Work out the finished part from the listing and answer in its coordinate system (mm). Coordinates: 2 decimals unless noted, no trailing zeros. Write each loop counter-clockwise with the first axis right and the second up, starting at its lowest first coordinate (ties: lowest second). Pieces come first, ordered by that corner, then holes. Notation, with made-up numbers: (69, -35.75) -> (103, -35.75) arc R16 cw to (103, -25.75) -> close; hole circle Ø6 at (47.5, 10). An arc over 180 degrees is marked (long way). Write each question's results on one line, items separated by ' | '. Start each with the question number.
from build123d import *

# Parameters (mm, degrees)
CROQUIS1_R              = 1.5
CROQUIS1_W              = 44
CROQUIS1_H              = 26
CROQUIS1_W_2            = 5
CROQUIS1_H_2            = 26.666666666
CROQUIS1_W_3            = 76.666666666
CROQUIS1_H_3            = 5
SALIENTE_EXTRUIR1_DEPTH = 5
CROQUIS2_R              = 4.15
CORTAR_EXTRUIR1_DEPTH   = 10
CROQUIS3_W              = 19
CROQUIS3_H              = 13
CORTAR_EXTRUIR2_DEPTH   = 10
CROQUIS4_R              = 4.15
CORTAR_EXTRUIR3_DEPTH   = 10
CROQUIS5_R              = 6
CORTAR_EXTRUIR4_DEPTH   = 10
CROQUIS7_W              = 87.958060954
CROQUIS7_H              = 14.714173765
SALIENTE_EXTRUIR2_DEPTH = 5


with BuildPart() as part:
    # Croquis1 → Saliente-Extruir1 (new body)
    with BuildSketch(Plane.XY):
        Polygon((5, 26.666666667), (5, 5), (76.666666667, 5), (153.333333333, 5), (225, 5), (225, 26.666666667), (225, 53.333333333), (225, 75), (153.333333333, 75), (76.666666667, 75), (5, 75), (5, 53.333333333), align=None)
        with Locations((30, 39)):
            Circle(CROQUIS1_R, mode=Mode.SUBTRACT)
        with Locations((83.04, 39)):
            Circle(CROQUIS1_R, mode=Mode.SUBTRACT)
        with Locations((56.52, 52)):
            Rectangle(CROQUIS1_W, CROQUIS1_H, mode=Mode.SUBTRACT)
        with Locations((30, 65)):
            Circle(CROQUIS1_R, mode=Mode.SUBTRACT)
        with Locations((83.04, 65)):
            Circle(CROQUIS1_R, mode=Mode.SUBTRACT)
        with Locations((227.5, 40)):
            Rectangle(CROQUIS1_W_2, CROQUIS1_H_2)
        with Locations((115, 2.5)):
            Rectangle(CROQUIS1_W_3, CROQUIS1_H_3)
        with Locations((2.5, 40)):
            Rectangle(CROQUIS1_W_2, CROQUIS1_H_2)
        with Locations((115, 77.5)):
            Rectangle(CROQUIS1_W_3, CROQUIS1_H_3)
    extrude(amount=SALIENTE_EXTRUIR1_DEPTH)

    # Croquis2 → Cortar-Extruir1 (cut)
    with BuildSketch(Plane.XY.offset(5)):
        with Locations((96.666666667, 20)):
            Circle(CROQUIS2_R)
        with Locations((116.666666667, 20)):
            Circle(CROQUIS2_R)
        with Locations((136.666666667, 20)):
            Circle(CROQUIS2_R)
    extrude(amount=-CORTAR_EXTRUIR1_DEPTH, mode=Mode.SUBTRACT)

    # Croquis3 → Cortar-Extruir2 (cut)
    with BuildSketch(Plane.XY.offset(5)):
        with Locations((34.5, 20.5)):
            Rectangle(CROQUIS3_W, CROQUIS3_H)
    extrude(amount=-CORTAR_EXTRUIR2_DEPTH, mode=Mode.SUBTRACT)

    # Croquis4 → Cortar-Extruir3 (cut)
    with BuildSketch(Plane.XY.offset(5)):
        with Locations((65, 20)):
            Circle(CROQUIS4_R)
        with Locations((80, 20)):
            Circle(CROQUIS4_R)
    extrude(amount=-CORTAR_EXTRUIR3_DEPTH, mode=Mode.SUBTRACT)

    # Croquis5 → Cortar-Extruir4 (cut)
    with BuildSketch(Plane.XY.offset(5)):
        with Locations((98.52, 50)):
            Circle(CROQUIS5_R)
        with Locations((120.52, 50)):
            Circle(CROQUIS5_R)
    extrude(amount=-CORTAR_EXTRUIR4_DEPTH, mode=Mode.SUBTRACT)

    # Croquis7 → Saliente-Extruir2 (add)
    with BuildSketch(Plane.XY.offset(5)):
        with Locations((100.697748768, 19.971943706)):
            Rectangle(CROQUIS7_W, CROQUIS7_H)
    extrude(amount=-SALIENTE_EXTRUIR2_DEPTH)


solid = part.part
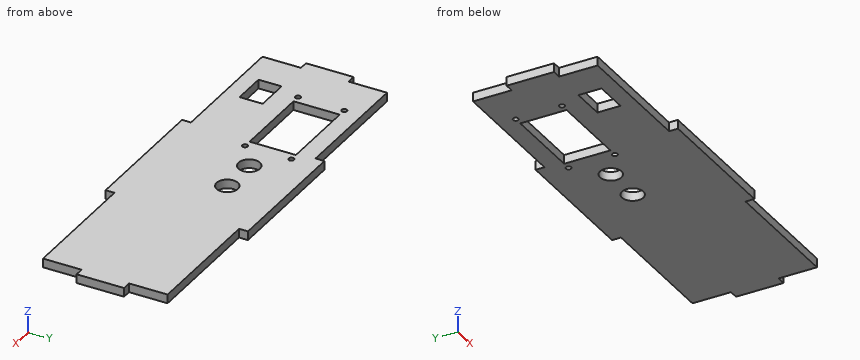
1. Find section A-A on x = 98.52. Give the vertices of the cut face in (y, z).
2. Find section C-C on x = 41.5. Give the vertices of the cut face in (y, z), and give its area (3 significant figures).
3. Given pin 1 Ø2.5 at (x, y) = (30, 65) entering from -Z; pin 2 Ø1.5 at (y, z) = (3, 1.5) entering from -X; pin 3 Ø1.5 at (y, z) = (20.5, 3.5) entering from -X; pin 4 Ø19 at (x, y) = (120.52, 50) entering from +Z, each flat-ended and moving along its own axis, determine where each tip first touches the part or whether it passes through.
4. Find section B-B on y = 50. Give the vertices of the cut face in (x, z).
5. Find the intervals of material crossed by L1, parallel to Y at x = 83.04, z = 1.4; L2, parallel to X at y = 15, z = 1.85; L3, parallel to Y at x = 98.52, z = 1, in increasing order.
6. Find section D-D on x = 74. Give the vertices of the cut face in (y, z), and give its area (3 significant figures).
Ans:
1) outline: (0, 0) -> (44, 0) -> (44, 5) -> (0, 5) -> close; (56, 0) -> (80, 0) -> (80, 5) -> (56, 5) -> close
2) outline: (5, 0) -> (14, 0) -> (14, 5) -> (5, 5) -> close; (27, 0) -> (39, 0) -> (39, 5) -> (27, 5) -> close; (65, 0) -> (75, 0) -> (75, 5) -> (65, 5) -> close | area: 155 mm²
3) pin 1: passes through | pin 2: stops at x = 76.67 | pin 3: stops at x = 5 | pin 4: stops at z = 5
4) outline: (0, 0) -> (34.52, 0) -> (34.52, 5) -> (0, 5) -> close; (78.52, 0) -> (92.52, 0) -> (92.52, 5) -> (78.52, 5) -> close; (104.52, 0) -> (114.52, 0) -> (114.52, 5) -> (104.52, 5) -> close; (126.52, 0) -> (230, 0) -> (230, 5) -> (126.52, 5) -> close
5) L1: y = 0 to 37.5, 40.5 to 63.5, 66.5 to 80 | L2: x = 5 to 25, 44 to 225 | L3: y = 0 to 44, 56 to 80
6) outline: (5, 0) -> (39, 0) -> (39, 5) -> (5, 5) -> close; (65, 0) -> (75, 0) -> (75, 5) -> (65, 5) -> close | area: 220 mm²
